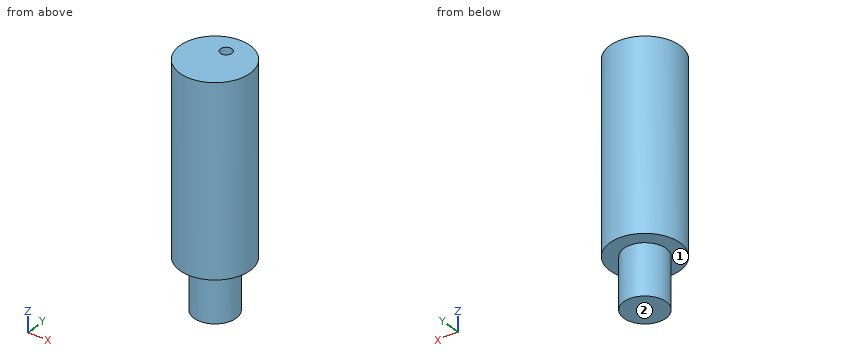
from build123d import *

# Parameters (mm, degrees)
F0_R     = 5.715
F1_DEPTH = 13.716
F2_R     = 9.525
F2_R_2   = 5.715
F3_DEPTH = 50.8
F4_R     = 1.564291
F5_DEPTH = 6.35


with BuildPart() as f1:
    # F0 (on Top) → F1 (new body)
    with BuildSketch(Plane.XY):
        Circle(F0_R)
    extrude(amount=F1_DEPTH)

    # F2 (on face) → F3 (join)
    with BuildSketch(Plane.XY.offset(13.716)):
        Circle(F2_R)
        Circle(F2_R_2, mode=Mode.SUBTRACT)
        Circle(F2_R_2)
    extrude(amount=F3_DEPTH)

    # F4 (on face) → F5 (cut)
    with BuildSketch(Plane.XY.offset(64.516)):
        with Locations((0, 4.160097)):
            Circle(F4_R)
    extrude(amount=-F5_DEPTH, mode=Mode.SUBTRACT)


solid = f1.part
Could you check a few things on this model? Use its own coordinates, in mm. Face numbers are marked on the shaded views. A direction names the side the tool comes from. Give positions to 0.01 mm unless a question says otherwise; leave off trailing zeros. Order: outer loops, then holes, each group sorted by start corner. A loop starts at its lowest first (then second) coordinate and runs counter-clockwise, first axis right, second up. Notation, with made-up numbers: (-4.5, 32) -> (-0.5, 32) arc R14 cw to (-0.5, 36) -> close; hole circle Ø3 at (-2, -17.5). An arc over 180 degrees is marked (long way). Return JSON: item names as keys, results as strings.
1. On a 3-axis mill with a long thin cutter (end or side, diameter ignored), from which of +Z, -Z, +X, -X, +Y, -Y can I reach the whole of each face in a straight line? I mean the marked faces 1 and 2. Say none if no direction works.
Answer list:
{"face 1": "-Z", "face 2": "-Z, +X, -X, +Y, -Y"}
2. Imagine slicing it at D-D on x = -4. List the corners of the cut face in (y, z) for me, then the cut area to 3 significant figures.
Answer list:
{"outline": "(-8.64, 13.72) -> (-4.08, 13.72) -> (-4.08, 0) -> (4.08, 0) -> (4.08, 13.72) -> (8.64, 13.72) -> (8.64, 64.52) -> (-8.64, 64.52) -> close", "area": "990 mm2"}
3. I need wall thicknesses on line 1 (Y direction, x = 0, z = 63.25) (3 decimals); line 2 (Z direction, x = 6.25, y = -2.25); line 3 (Y direction, x = 0.5, z = 31.5). Which ranges of each line are inside material? Lowest first, please. Write a range as from..to.
Answer list:
{"line 1": "y = -9.525..2.596, 5.724..9.525", "line 2": "z = 13.72..64.52", "line 3": "y = -9.51..9.51"}
4. For pin 1 Ø2 at (x, z) = (-7, 57) entering from +Y; pin 2 Ø4 at (y, z) = (-6.5, 40) entering from -X (3 decimals); pin 3 Ø1.5 at (x, y) = (-1.5, 7.5) entering from -Z, each with a flat end and sliding along its axis, tell me the tip position at first contact or that it passes through.
Answer list:
{"pin 1": "stops at y = 7.4", "pin 2": "stops at x = -8.395", "pin 3": "stops at z = 13.72"}
5. Imagine slicing it at C-C on z = 11. List the corners of the cut face in (x, y) for me (3 decimals), then the cut area to 3 significant figures.
Answer list:
{"outline": "circle Ø11.43 at (0, 0)", "area": "103 mm2"}
6. Imagine slicing it at A-A on x = 0. List the corners of the cut face in (y, z) for me (3 decimals).
Answer list:
{"outline": "(-9.525, 13.716) -> (-5.715, 13.716) -> (-5.715, 0) -> (5.715, 0) -> (5.715, 13.716) -> (9.525, 13.716) -> (9.525, 64.516) -> (5.724, 64.516) -> (5.724, 58.166) -> (2.596, 58.166) -> (2.596, 64.516) -> (-9.525, 64.516) -> close"}
7. Imagine slicing it at B-B on y = 0. List the corners of the cut face in (x, z) for me (3 decimals).
Answer list:
{"outline": "(-9.525, 13.716) -> (-5.715, 13.716) -> (-5.715, 0) -> (5.715, 0) -> (5.715, 13.716) -> (9.525, 13.716) -> (9.525, 64.516) -> (-9.525, 64.516) -> close"}
